Autodesk Inventor part; units mm, degrees
ref_plane "YZ Plane" through (0, 0, 0) normal (1, 0, 0) x (0, 1, 0)
ref_plane "XZ Plane" through (0, 0, 0) normal (0, 1, 0) x (-1, 0, 0)
ref_plane "XY Plane" through (0, 0, 0) normal (0, 0, 1) x (1, 0, 0)
sketch "Esboço1" plane through (0, 0, 0) normal (0, 1, 0) x (-1, 0, 0)
  arc A0 (-350, 0) -> (-247.4874, -247.4874) centre (0, 0) ccw
  arc A1 (-400, 0) -> (-282.8427, -282.8427) centre (0, 0) ccw
  circle A2 centre (0, 0) radius 400
  circle A3 centre (0, 0) radius 350
  line L0 (0, 0) -> (-407.9373, -407.9373)
  line L1 (0, 0) -> (-1224.3013, 0) construction
  line L2 (-350, 0) -> (-400, 0)
  point P0 (-282.8427, -282.8427)
  point P1 (-247.4874, -247.4874)
  dimension "d27" = 700
  dimension "d28" = 800
  dimension "d87" = 45
extrude "Extrusão1" add sketch "Esboço1" along normal blind 6 contours A0 L0 A1 L2
sketch "Esboço5" plane through (0, 6, 0) normal (0, 1, 0) x (1, 0, 0)
  arc A0 (400, 0) -> (282.8427, 282.8427) centre (0, 0) ccw
  circle A1 centre (0, 0) radius 400
  circle A2 centre (0, 0) radius 350
  line L0 (0, 0) -> (356.9788, 299.5408)
  line L1 (282.8427, 282.8427) -> (247.4874, 247.4874)
  line L2 (282.8427, 282.8427) -> (272.2361, 272.2361)
  line L3 (272.2361, 272.2361) -> (258.094, 258.094)
  line L4 (258.094, 258.094) -> (247.4874, 247.4874)
  line L5 (306.4178, 257.115) -> (292.629, 245.5449)
  line L6 (292.629, 245.5449) -> (281.9044, 236.5458)
  line L7 (281.9044, 236.5458) -> (268.1156, 224.9757)
  line L8 (258.094, 258.094) -> (281.9044, 236.5458)
  line L9 (272.2361, 272.2361) -> (292.629, 245.5449)
  point P0 (306.4178, 257.115)
  dimension "d88" = -5
  dimension "d89" = 15
  dimension "d90" = 20
  dimension "d91" = 18
  dimension "d92" = 14
extrude "Extrusão5" cut sketch "Esboço5" against normal up to surface (6 mm away) contours L0 L9 L1 A0 | L0 A2 L1 L8
sketch "Esboço6" plane through (0, 6, 0) normal (0, 1, 0) x (1, 0, 0)
  arc A0 (400, 0) -> (306.4178, 257.115) centre (0, 0) ccw
  circle A1 centre (0, 0) radius 400
  arc A2 (350, 0) -> (224.9757, 268.1156) centre (0, 0) ccw
  circle A3 centre (0, 0) radius 350
  line L0 (0, 0) -> (512.6153, 44.848)
  line L1 (350, 0) -> (400, 0)
  line L2 (350, 0) -> (368, 0)
  line L3 (368, 0) -> (382, 0)
  line L4 (382, 0) -> (400, 0)
  line L5 (348.6681, 30.5045) -> (363.6111, 31.8118)
  line L6 (363.6111, 31.8118) -> (383.535, 33.555)
  line L7 (383.535, 33.555) -> (398.4779, 34.8623)
  line L8 (368, 0) -> (363.6111, 31.8118)
  line L9 (382, 0) -> (383.535, 33.555)
  point P0 (257.115, 306.4178)
  dimension "d93" = -5
  dimension "d94" = 18
  dimension "d95" = 14
  dimension "d96" = 15
  dimension "d97" = 20
extrude "Extrusão6" cut sketch "Esboço6" against normal up to surface (6 mm away) contours L1 L8 L0 L9
properties part number "base"
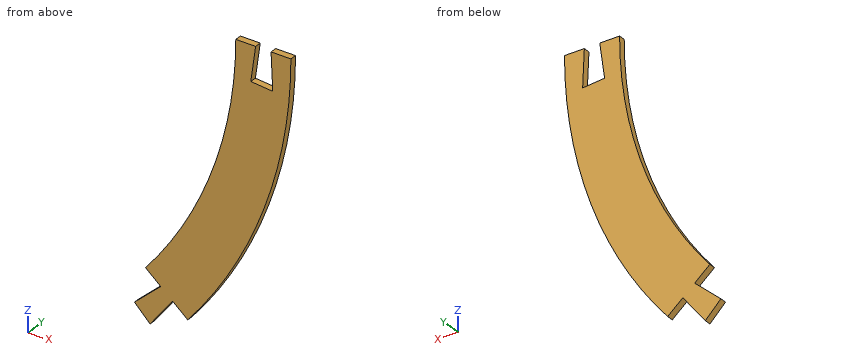
Could you check a few things on this model? Use its own coordinates, in mm. Round coordinates to 2 decimals unless told otherwise and drop trailing zeros. Write each loop counter-clockwise with the first axis right and the second up, starting at its lowest first coordinate (ties: lowest second). Pieces come first, ordered by that corner, then holes. Notation, with made-up numbers: (2.25, -19) -> (35.25, -19) arc R18 ccw to (35.25, 15) -> close; hole circle Ø3 at (66, 83.5). An arc over 180 degrees is marked (long way). Use a Markdown table: item, result.
1. For pin 1 Ø3 at (y, z) = (0.5, -215.5) entering from -X; pin 2 Ø3 at (x, y) = (362.5, 4.5) entering from -Z, each with a flat end and sliding along its axis, tell me the tip position at first contact or that it passes through.
Answer key:
| item | result |
|---|---|
| pin 1 | stops at x = 274.61 |
| pin 2 | stops at z = -172.28 |
2. Please list where these lines run through material, in increasing order: probe 1 along Z at (x, y) = (279, 5.6); probe 2 along X at (y, z) = (1.8, -101); probe 3 along X at (y, z) = (3, -123).
Answer key:
| item | result |
|---|---|
| probe 1 | z = -263.38 to -239.17, -234.11 to -211.33 |
| probe 2 | x = 335.11 to 387.04 |
| probe 3 | x = 327.68 to 380.62 |
3. If we section it at C-C (x = 388.5): List the corners of the cut face in (y, z) for me, then the cut area to 3 significant figures.
Answer key:
| item | result |
|---|---|
| outline | (0, -95.22) -> (6, -95.22) -> (6, 0) -> (0, 0) -> close |
| area | 571 mm^2 |
4. If we section it at A-A (z = -22): List the corners of the cut face in (x, y) for me.
Answer key:
| item | result |
|---|---|
| outline | (349.31, 0) -> (364.96, 0) -> (364.96, 6) -> (349.31, 6) -> close; (383.01, 0) -> (399.39, 0) -> (399.39, 6) -> (383.01, 6) -> close |
5. If we section it at B-B (y = 3.45): List the corners of the cut face in (x, z) for me (1 decimal).
Answer key:
| item | result |
|---|---|
| outline | (258.1, -258.1) -> (272.2, -272.2) -> (292.6, -245.5) -> (306.4, -257.1) arc R400 ccw to (400, 0) -> (382, 0) -> (383.5, -33.6) -> (363.6, -31.8) -> (368, 0) -> (350, 0) arc R350 cw to (268.1, -225) -> (281.9, -236.5) -> close |
6. If we section it at D-D (z = -167.5): List the corners of the cut face in (x, y) for me, then the cut area to 3 significant figures.
Answer key:
| item | result |
|---|---|
| outline | (307.32, 0) -> (363.24, 0) -> (363.24, 6) -> (307.32, 6) -> close |
| area | 336 mm^2 |
